Autodesk Inventor part; units mm, degrees
ref_plane "YZ Plane" through (0, 0, 0) normal (1, 0, 0) x (0, 1, 0)
ref_plane "XZ Plane" through (0, 0, 0) normal (0, 1, 0) x (-1, 0, 0)
ref_plane "XY Plane" through (0, 0, 0) normal (0, 0, 1) x (1, 0, 0)
sketch "Sketch1" plane through (0, 0, 0) normal (1, 0, 0) x (0, 1, 0)
  line L0 (31.75, -180) -> (-31.75, -180)
  line L1 (-31.75, -180) -> (-31.75, 180)
  line L2 (-31.75, 180) -> (31.75, 180)
  line L3 (31.75, 180) -> (31.75, -180)
  line L4 (31.75, -180) -> (-31.75, 180) construction
  line L5 (-31.75, -180) -> (31.75, 180) construction
  line L6 (-31.75, 0) -> (31.75, 0) construction
  line L7 (0, 180) -> (0, -180) construction
  line L8 (24, -88) -> (-24, -88) construction
  line L9 (24, -117) -> (-24, -117) construction
  line L10 (16.75, -153) -> (-16.75, -153) construction
  line L11 (24, 88) -> (-24, 88) construction
  line L12 (24, 117) -> (-24, 117) construction
  line L13 (16.75, 153) -> (-16.75, 153) construction
  line L14 (24, -117) -> (24, -88) construction
  arc A0 (-6.8516, 158.566) -> (6.8516, 158.566) centre (0, 160) ccw
  line L15 (-15, 197.5) -> (15, 197.5)
  line L16 (15, 197.5) -> (6.8516, 158.566)
  line L17 (-15, 197.5) -> (-6.8516, 158.566)
  arc A1 (6.8516, -158.566) -> (-6.8516, -158.566) centre (0, -160) ccw
  line L18 (-15, -197.5) -> (15, -197.5)
  line L19 (15, -197.5) -> (6.8516, -158.566)
  line L20 (-15, -197.5) -> (-6.8516, -158.566)
  point P0 (0, 0)
  point P1 (-20.25, 0)
  point P2 (20.25, 0)
  point P3 (0, 153)
  point P4 (-11.3374, -180)
  point P5 (11.3374, -180)
  point P6 (11.3374, 180)
  point P7 (-11.3374, 180)
  point P8 (0, 58.5)
  point P9 (0, -58.5)
  dimension "d0" = 63.5
  dimension "d1" = 360
  dimension "d2" = 40.5
  dimension "d3" = 176
  dimension "d4" = 29
  dimension "d5" = 48
  dimension "d6" = 33.5
  dimension "d7" = 306
  dimension "d8" = 30
  dimension "d9" = 37.5
  dimension "d10" = 14
  dimension "d11" = 320
  dimension "d21" = 117
extrude "Extrusion1" add sketch "Sketch1" along normal blind 5 contours L0 L19 A1 L20 L1 L2 L17 A0 L16 L3
hole "Hole1" at (0, -20.25, 0) at (0, 20.25, 0) at (0, 24, -88) at (0, 24, -117) at (0, 16.75, -153) at (0, -24, -88) at (0, -24, -117) at (0, -16.75, -153) at (0, 24, 88) at (0, 24, 117) at (0, 16.75, 153) at (0, -16.75, 153) at (0, -24, 117) at (0, -24, 88) at (0, 0, 160) at (0, 0, -160) direction (1, 0, 0) diameter 6 end through all
hole "Hole2" at (0, 0, 58.5) at (0, 0, -58.5) direction (1, 0, 0) diameter 6.647 end through all
fillet "Fillet1" radius 5 8 edges at (2.5, 31.75, 180) (2.5, -31.75, 180) (2.5, 31.75, -180) (2.5, 11.3374, -180) (2.5, -11.3374, -180) (2.5, -31.75, -180) (2.5, -11.3374, 180) (2.5, 11.3374, 180)
properties part number "ServoMotorsInitialPositioningFrame" material "Aluminum 7075"
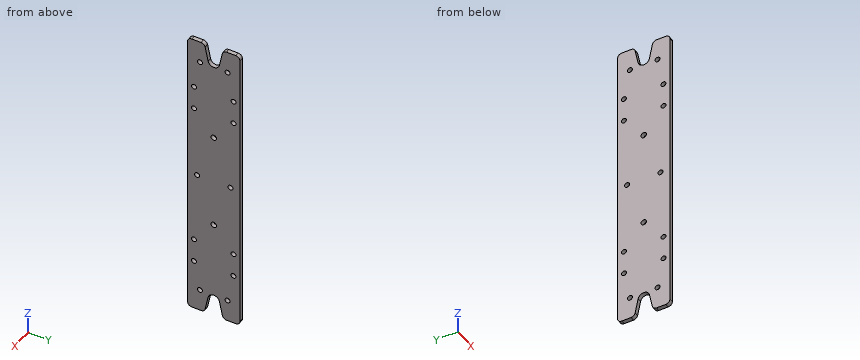
Check sheet for the modelled part. Datum: model origin and axes. Units: mm. Coordinates: 2 decimals unless noted, no trailing zeros. Loops run counter-clockwise (first coordinate to the right, second up) from the corner with the lowest first, then second, coordinate; pieces in that order, holes last. Notation, with made-up numbers: (1, 26) -> (24, 26) arc R25 ccw to (24, 52) -> close; hole circle Ø6 at (2.25, 80.25). An arc over 180 degrees is marked (long way). Write item = value, one per line. Start each with the question number.
1. Material ranges on line 1 (Y direction, x = 3.3, z = -88); line 2 (Z direction, x = 2.5, y = 16.75); line 3 (Z direction, x = 3.9, y = -24), recorded low to high.
2. Section check B-B on z = 88. Record the cut outline in (x, y), then the cut area to 4 significant figures.
3. Section check C-C on x = 4. Give the number of separate pieces and of enclosed holes in the cut face, then the cut area to 3 significant figures.
4. Section check A-A on y = 0. Record the cut outline in (x, z), then the cut area to 3 significant figures.
Responses:
q1.line_1 = -31.75 to -27, -21 to 21, 27 to 31.75
q1.line_2 = -180 to -156, -150 to 150, 156 to 180
q1.line_3 = -180 to -120, -114 to -91, -85 to 85, 91 to 114, 120 to 180
q2.outline = (0, -31.75) -> (5, -31.75) -> (5, -27) -> (0, -27) -> close; (0, -21) -> (5, -21) -> (5, 21) -> (0, 21) -> close; (0, 27) -> (5, 27) -> (5, 31.75) -> (0, 31.75) -> close
q2.area = 257.5 mm2
q3.separate_pieces = 1
q3.enclosed_holes = 16
q3.area = 21,500 mm2
q4.outline = (0, -153) -> (5, -153) -> (5, -61.82) -> (0, -61.82) -> close; (0, -55.18) -> (5, -55.18) -> (5, 55.18) -> (0, 55.18) -> close; (0, 61.82) -> (5, 61.82) -> (5, 153) -> (0, 153) -> close
q4.area = 1,460 mm2
